from build123d import *

# Parameters (mm, degrees)
ESQUISSE1_W             = 111.5
ESQUISSE1_H             = 13
BOSS_EXTRU_1_DEPTH      = 1.5
ESQUISSE2_W             = 111.5
ESQUISSE2_H             = 1.5
BOSS_EXTRU_2_DEPTH      = 8.4
ESQUISSE4_R             = 1.4
ENL_V_MAT_EXTRU_1_DEPTH = 20


with BuildPart() as part:
    # Esquisse1 → Boss.-Extru.1 (new body)
    with BuildSketch(Plane(origin=(0, 0, 0), x_dir=(1, 0, 0), z_dir=(0, 1, 0))):
        with Locations((55.75, 6.5)):
            Rectangle(ESQUISSE1_W, ESQUISSE1_H)
    extrude(amount=BOSS_EXTRU_1_DEPTH)

    # Esquisse2 → Boss.-Extru.2 (add)
    with BuildSketch(Plane(origin=(0, 1.5, 0), x_dir=(1, 0, 0), z_dir=(0, 1, 0))):
        with Locations((55.75, 12.25)):
            Rectangle(ESQUISSE2_W, ESQUISSE2_H)
        with Locations((55.75, 0.75)):
            Rectangle(ESQUISSE2_W, ESQUISSE2_H)
    extrude(amount=BOSS_EXTRU_2_DEPTH)

    # Esquisse4 → Enlèv. mat.-Extru.1 (cut)
    with BuildSketch(Plane.XY):
        with Locations((37, 5.4)):
            Circle(ESQUISSE4_R)
        with Locations((55, 5.4)):
            Circle(ESQUISSE4_R)
        with Locations((73, 5.4)):
            Circle(ESQUISSE4_R)
        with Locations((15.200278481, 5.4)):
            Circle(ESQUISSE4_R)
        with Locations((98.200278481, 5.4)):
            Circle(ESQUISSE4_R)
    extrude(amount=-ENL_V_MAT_EXTRU_1_DEPTH, mode=Mode.SUBTRACT)


solid = part.part
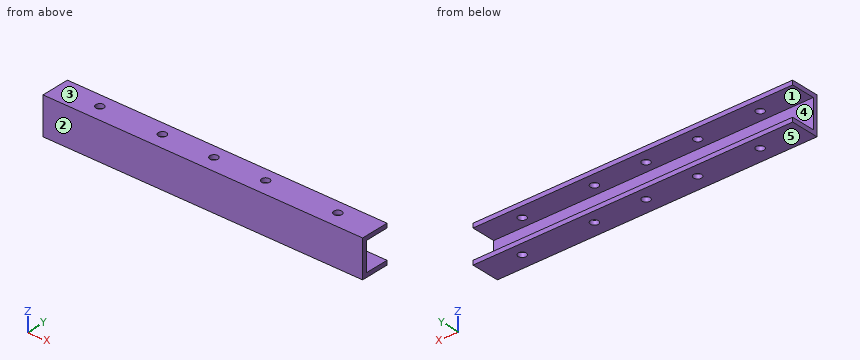
The listing builds one solid part. Answer for the finished solid, in the listing's coordinates (mm). Face numbers are marked on the shaded views. A direction names the side the tool comes from. Coordinates: 2 decimals unless noted, no trailing zeros. Write each loop counter-clockwise with the first axis right and the second up, starting at its lowest first coordinate (ties: lowest second). Pieces come first, ordered by that corner, then holes. Notation, with made-up numbers: (39, -4) - (58, -4) arc R24 cw to (58, 6) - close; hole circle Ø1 at (20.25, 0.5). An arc over 180 degrees is marked (long way). Answer as CSV lines item,"result".
1. Find section C-C (x = 79). Give the vertices of the cut face in (y, z).
Computed values:
outline,"(0, -13) - (9.9, -13) - (9.9, -11.5) - (1.5, -11.5) - (1.5, -1.5) - (9.9, -1.5) - (9.9, 0) - (0, 0) - close"
2. Find section A-A (x = 55). Give the vertices of the cut face in (y, z), plus the area to 3 significant figures.
Computed values:
outline,"(0, -13) - (4, -13) - (4, -11.5) - (1.5, -11.5) - (1.5, -1.5) - (4, -1.5) - (4, 0) - (0, 0) - close; (6.8, -13) - (9.9, -13) - (9.9, -11.5) - (6.8, -11.5) - close; (6.8, -1.5) - (9.9, -1.5) - (9.9, 0) - (6.8, 0) - close"
area,"36.3 mm²"
3. Straight lines are drawn through the part: line 1 (Z direction, x = 56, y = 6.75); line 2 (Y direction, x = 73, z = -0.9); line 3 (Y direction, x = 22.5, z = -6.25). For each, find the intervals that lie inside material, in ascending order. Write a range as [from, to].
Computed values:
line 1,"z = [-13, -11.5], [-1.5, 0]"
line 2,"y = [0, 4], [6.8, 9.9]"
line 3,"y = [0, 1.5]"
4. Find section D-D (z = -8.5). Give the vertices of the cut face in (x, y).
Computed values:
outline,"(0, 0) - (111.5, 0) - (111.5, 1.5) - (0, 1.5) - close"
5. Determine the mould class of the marked faces 3, 4 and 5 for opening direction Z: +Z half, -Z half, draft (parallel to the pull), parting line (faces both ways), or undercut.
Computed values:
face 3,"+Z half"
face 4,"undercut"
face 5,"-Z half"
6. A tool of negligible diameter and unlimited length cuts with its end or side. For the marked faces 1 and 2, from which of +Z, -Z, +X, -X, +Y, -Y can it reach the whole face along a straight path? Write none if from no direction.
Computed values:
face 1,"+X, -X, +Y"
face 2,"+Z, -Z, +X, -X, -Y"
7. Given P1, Ø2.5, axis at x = 55, y = 5.4, coming from the -Z side; P2, Ø1.5, axis at x = 90, z = -2.5, coming from the -Y side; P3, Ø3, axis at x = 32.5, z = -9, coming from the +Y side, each flat-ended and moving along its own axis, determine where each tip first touches the part or whether it passes through.
Computed values:
P1,"passes through"
P2,"stops at y = 0"
P3,"stops at y = 1.5"
8. Find section B-B (y = 8.75). Give the vertices of the cut face in (x, z), plus the area to 4 significant figures.
Computed values:
outline,"(0, -13) - (111.5, -13) - (111.5, -11.5) - (0, -11.5) - close; (0, -1.5) - (111.5, -1.5) - (111.5, 0) - (0, 0) - close"
area,"334.5 mm²"
